Geometry: final body of the model. Coordinates: model frame, mm. Give positions to 0.01 mm unless a question says otherwise; leave off trailing zeros. Loops run counter-clockwise (first coordinate to the right, second up) from the corner with the lowest first, then second, coordinate; pieces in that order, holes last. Notation, with made-up numbers: (85, 77.5) -> (110, 77.5) arc R13 cw to (110, 91.5) -> close; hole circle Ø8 at (74, 46). An arc over 180 degrees is marked (long way). One line per item, written item: value. Start each with the question number.
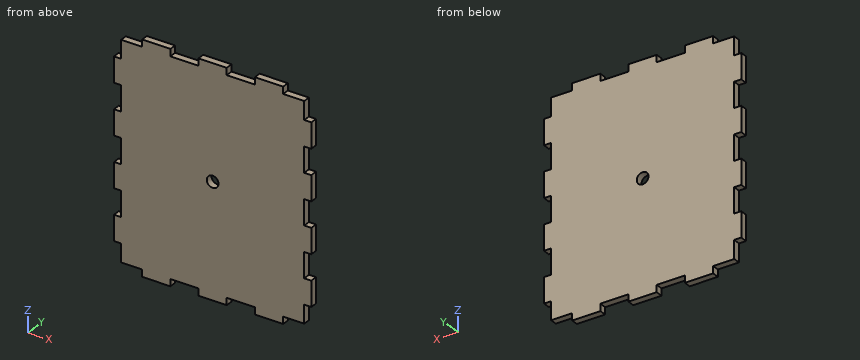
from build123d import *

# Parameters (mm, degrees)
ESBO_O1_W                = 84
ESBO_O1_H                = 97
RESSALTO_EXTRUS_O1_DEPTH = 3
ESBO_O2_W                = 3
ESBO_O2_H                = 10.777777778
CORTE_EXTRUS_O4_DEPTH    = 3
CORTE_EXTRUS_O9_REACH    = 66.228
ESBO_O5_W                = 12
ESBO_O5_H                = 3
CORTE_EXTRUS_O10_REACH   = 66.228
ESBO_O6_R                = 2.5


with BuildPart() as part:
    # Esboço1 → Ressalto-extrusão1 (new body)
    with BuildSketch(Plane(origin=(0, 0, 0), x_dir=(1, 0, 0), z_dir=(0, 1, 0))):
        Rectangle(ESBO_O1_W, ESBO_O1_H)
    extrude(amount=RESSALTO_EXTRUS_O1_DEPTH)

    # Esboço2 → Corte-extrusão4 (cut)
    with BuildSketch(Plane.XZ):
        with Locations((-40.5, -43.111111111)):
            Rectangle(ESBO_O2_W, ESBO_O2_H)
        with Locations((40.5, -43.111111111)):
            Rectangle(ESBO_O2_W, ESBO_O2_H)
        with Locations((40.5, -21.551111111)):
            Rectangle(ESBO_O2_W, ESBO_O2_H)
        with Locations((40.5, 0.008888889)):
            Rectangle(ESBO_O2_W, ESBO_O2_H)
        with Locations((40.5, 21.568888889)):
            Rectangle(ESBO_O2_W, ESBO_O2_H)
        with Locations((40.5, 43.128888889)):
            Rectangle(ESBO_O2_W, ESBO_O2_H)
        with Locations((-40.5, -21.551111111)):
            Rectangle(ESBO_O2_W, ESBO_O2_H)
        with Locations((-40.5, 0.008888889)):
            Rectangle(ESBO_O2_W, ESBO_O2_H)
        with Locations((-40.5, 21.568888889)):
            Rectangle(ESBO_O2_W, ESBO_O2_H)
        with Locations((-40.5, 43.128888889)):
            Rectangle(ESBO_O2_W, ESBO_O2_H)
    extrude(amount=-CORTE_EXTRUS_O4_DEPTH, mode=Mode.SUBTRACT)

    # Esboço5 → Corte-extrusão9 (cut, up to next)
    with BuildSketch(Plane(origin=(0, 0, 0), x_dir=(1, 0, 0), z_dir=(0, 1, 0)), mode=Mode.PRIVATE) as corte_extrus_o9_sk1:
        with Locations((-36, 47)):
            Rectangle(ESBO_O5_W, ESBO_O5_H)
    corte_extrus_o9_tool1 = extrude(corte_extrus_o9_sk1.sketch, amount=CORTE_EXTRUS_O9_REACH, mode=Mode.PRIVATE) & part.part
    # Esboço5 → Corte-extrusão9 (cut, up to next)
    with BuildSketch(Plane(origin=(0, 0, 0), x_dir=(1, 0, 0), z_dir=(0, 1, 0)), mode=Mode.PRIVATE) as corte_extrus_o9_sk2:
        with Locations((-36, -47)):
            Rectangle(ESBO_O5_W, ESBO_O5_H)
    corte_extrus_o9_tool2 = extrude(corte_extrus_o9_sk2.sketch, amount=CORTE_EXTRUS_O9_REACH, mode=Mode.PRIVATE) & part.part
    # Esboço5 → Corte-extrusão9 (cut, up to next)
    with BuildSketch(Plane(origin=(0, 0, 0), x_dir=(1, 0, 0), z_dir=(0, 1, 0)), mode=Mode.PRIVATE) as corte_extrus_o9_sk3:
        with Locations((36, -47)):
            Rectangle(ESBO_O5_W, ESBO_O5_H)
    corte_extrus_o9_tool3 = extrude(corte_extrus_o9_sk3.sketch, amount=CORTE_EXTRUS_O9_REACH, mode=Mode.PRIVATE) & part.part
    # Esboço5 → Corte-extrusão9 (cut, up to next)
    with BuildSketch(Plane(origin=(0, 0, 0), x_dir=(1, 0, 0), z_dir=(0, 1, 0)), mode=Mode.PRIVATE) as corte_extrus_o9_sk4:
        with Locations((36, 47)):
            Rectangle(ESBO_O5_W, ESBO_O5_H)
    corte_extrus_o9_tool4 = extrude(corte_extrus_o9_sk4.sketch, amount=CORTE_EXTRUS_O9_REACH, mode=Mode.PRIVATE) & part.part
    # Esboço5 → Corte-extrusão9 (cut, up to next)
    with BuildSketch(Plane(origin=(0, 0, 0), x_dir=(1, 0, 0), z_dir=(0, 1, 0)), mode=Mode.PRIVATE) as corte_extrus_o9_sk5:
        with Locations((-12, -47)):
            Rectangle(ESBO_O5_W, ESBO_O5_H)
    corte_extrus_o9_tool5 = extrude(corte_extrus_o9_sk5.sketch, amount=CORTE_EXTRUS_O9_REACH, mode=Mode.PRIVATE) & part.part
    # Esboço5 → Corte-extrusão9 (cut, up to next)
    with BuildSketch(Plane(origin=(0, 0, 0), x_dir=(1, 0, 0), z_dir=(0, 1, 0)), mode=Mode.PRIVATE) as corte_extrus_o9_sk6:
        with Locations((12, -47)):
            Rectangle(ESBO_O5_W, ESBO_O5_H)
    corte_extrus_o9_tool6 = extrude(corte_extrus_o9_sk6.sketch, amount=CORTE_EXTRUS_O9_REACH, mode=Mode.PRIVATE) & part.part
    # Esboço5 → Corte-extrusão9 (cut, up to next)
    with BuildSketch(Plane(origin=(0, 0, 0), x_dir=(1, 0, 0), z_dir=(0, 1, 0)), mode=Mode.PRIVATE) as corte_extrus_o9_sk7:
        with Locations((-12, 47)):
            Rectangle(ESBO_O5_W, ESBO_O5_H)
    corte_extrus_o9_tool7 = extrude(corte_extrus_o9_sk7.sketch, amount=CORTE_EXTRUS_O9_REACH, mode=Mode.PRIVATE) & part.part
    # Esboço5 → Corte-extrusão9 (cut, up to next)
    with BuildSketch(Plane(origin=(0, 0, 0), x_dir=(1, 0, 0), z_dir=(0, 1, 0)), mode=Mode.PRIVATE) as corte_extrus_o9_sk8:
        with Locations((12, 47)):
            Rectangle(ESBO_O5_W, ESBO_O5_H)
    corte_extrus_o9_tool8 = extrude(corte_extrus_o9_sk8.sketch, amount=CORTE_EXTRUS_O9_REACH, mode=Mode.PRIVATE) & part.part
    add(corte_extrus_o9_tool1.solids().sort_by_distance((-36, 0, -47))[0], mode=Mode.SUBTRACT)
    add(corte_extrus_o9_tool2.solids().sort_by_distance((-36, 0, 47))[0], mode=Mode.SUBTRACT)
    add(corte_extrus_o9_tool3.solids().sort_by_distance((36, 0, 47))[0], mode=Mode.SUBTRACT)
    add(corte_extrus_o9_tool4.solids().sort_by_distance((36, 0, -47))[0], mode=Mode.SUBTRACT)
    add(corte_extrus_o9_tool5.solids().sort_by_distance((-12, 0, 47))[0], mode=Mode.SUBTRACT)
    add(corte_extrus_o9_tool6.solids().sort_by_distance((12, 0, 47))[0], mode=Mode.SUBTRACT)
    add(corte_extrus_o9_tool7.solids().sort_by_distance((-12, 0, -47))[0], mode=Mode.SUBTRACT)
    add(corte_extrus_o9_tool8.solids().sort_by_distance((12, 0, -47))[0], mode=Mode.SUBTRACT)

    # Esboço6 → Corte-extrusão10 (cut, up to next)
    with BuildSketch(Plane.XZ, mode=Mode.PRIVATE) as corte_extrus_o10_sk1:
        with Locations(Location((0, 0, 0), (0, 0, 270))):
            Circle(ESBO_O6_R)
    corte_extrus_o10_tool1 = extrude(corte_extrus_o10_sk1.sketch, amount=-CORTE_EXTRUS_O10_REACH, mode=Mode.PRIVATE) & part.part
    add(corte_extrus_o10_tool1.solids().sort_by_distance((0, 0, 0))[0], mode=Mode.SUBTRACT)


solid = part.part
Item 1: Pin query (flat end, axial travel): pin 1 (0.9 mm diameter, centred on y = 1.5, z = 47, fed in from +X); pin 2 (0.9 mm diameter, centred on y = 1.5, z = 47.5, fed in from -X); pin 3 (1.5 mm diameter, centred on x = 40.5, y = 1, fed in from +Z). Return the tip coordinate at first contact, or that it passes through.
Item 2: Section C-C, the plane x = -15. Output: boundary loops of the cut face in (y, z), then the cut area to 3 significant figures.
Item 3: Ray query, line 1 along X through (y, z) = (2.15, 0); line 2 along Z through (x, y) = (-13.5, 1.6); line 3 along X through (y, z) = (2.4, -23.5). Return the intervals inside material, ascending. Write a range as [from, to].
Item 4: Section B-B, the plane x = 0. Output: boundary loops of the cut face in (y, z).
Item 5: Section A-A, the plane z = 0. Output: boundary loops of the cut face in (x, y), then the cut area to 3 significant figures.
Geometry check:
1. pin 1: stops at x = 30
1. pin 2: stops at x = -30
1. pin 3: stops at z = 37.74
2. outline: (0, -45.5) -> (3, -45.5) -> (3, 45.5) -> (0, 45.5) -> close
2. area: 273 mm2
3. line 1: x = [-39, -2.5], [2.5, 39]
3. line 2: z = [-45.5, 45.5]
3. line 3: x = [-39, 39]
4. outline: (0, -48.5) -> (3, -48.5) -> (3, -2.5) -> (0, -2.5) -> close; (0, 2.5) -> (3, 2.5) -> (3, 48.5) -> (0, 48.5) -> close
5. outline: (-39, 0) -> (-2.5, 0) -> (-2.5, 3) -> (-39, 3) -> close; (2.5, 0) -> (39, 0) -> (39, 3) -> (2.5, 3) -> close
5. area: 219 mm2
